from build123d import *

# Parameters (mm, degrees)
SKETCH_1_R               = 49
SKETCH_1_R_2             = 43
EXTRUDE_1_DEPTH          = 7.9
SKETCH_3_R               = 49
SKETCH_3_R_2             = 40.2
EXTRUDE_3_DEPTH          = 2
HOLE_WIZARD_M3_1_D       = 2.5
PATTERN_CIRCULAR_1_COUNT = 12


with BuildPart() as part:
    # 草图1 → 凸台-拉伸1 (new body)
    with BuildSketch(Plane.XY):
        Circle(SKETCH_1_R)
        Circle(SKETCH_1_R_2, mode=Mode.SUBTRACT)
    extrude(amount=EXTRUDE_1_DEPTH)

    # 草图3 → 凸台-拉伸3 (add)
    with BuildSketch(Plane.XY.offset(7.9)):
        Circle(SKETCH_3_R)
        Circle(SKETCH_3_R_2, mode=Mode.SUBTRACT)
    extrude(amount=EXTRUDE_3_DEPTH)

    # M3 螺纹孔1 (through all)
    with Locations(Plane(origin=(0, 0, 0), x_dir=(-1, 0, 0), z_dir=(0, 0, -1))):
        with Locations((0, 46)):
            hole_wizard_m3_1 = Hole(HOLE_WIZARD_M3_1_D / 2)

    # 阵列(圆周)1: M3 螺纹孔1 ×12 about axis
    pattern_circular_1_axis = Axis((0, 0, 0), (0, 0, 1))
    for i in range(1, PATTERN_CIRCULAR_1_COUNT):
        add(hole_wizard_m3_1.rotate(pattern_circular_1_axis, i * 360 / PATTERN_CIRCULAR_1_COUNT), mode=Mode.SUBTRACT)


solid = part.part
Geometry check sheet. Reference: the model listing, model coordinates, mm. A direction names the side the tool comes from. Round coordinates to 2 decimals unless told otherwise and drop trailing zeros. Order: outer loops, then holes, each group sorted by start corner. A loop starts at its lowest first (then second) coordinate and runs counter-clockwise, first axis right, second up. Notation, with made-up numbers: M -1.75,66 L 56.25,66 A22 cw 56.25,91 Z; hole C 45,-6.5 d3. An arc over 180 degrees is marked long. Answer in a Markdown table with one row per item. Add a question column.
Item 1: Material ranges on L1, parallel to Y at x = 0, z = 2.5; L2, parallel to Y at x = -1, z = 4.75; L3, parallel to X at y = 45, z = 4.75, recorded low to high. Write a range as [from, to].
Item 2: Sectioned sample at C-C, the plane y = -27. Enter the section's corners in (x, z), plus the area to 3 significant figures.
Item 3: Set-up check for faces 1 (the face through (-5.598, 42.634, 3.895)), 2 (the face through (24.11, -39.26, 5.02)): record each of +Z, -Z, +X, -X, +Y, -Y from which the full face is reachable in a straight line by a thin tool's end or side.
Item 4: Draft check along X on faces 3 (the face through (-0.16, 47.24, 5.02)), 4 (the face through (26.34, 41.32, 4.88)), 5 (the face through (-3.9, 40.2, 9.9)). Enter one of: released by +X, released by -X, zero draft, split by the parting line, or undercut.
Item 5: Sectioned sample at D-D, the plane x = -15.5. Enter the section's corners in (y, z), plus the area to 3 significant figures.
Item 6: Sectioned sample at A-A, the plane y = 0. Enter the section's corners in (x, z), plus the area to 3 significant figures.
Item 7: Depth check by flat-ended pin: pin 1 Ø2 at (x, y) = (0, 46) entering from -Z; pin 2 Ø1.5 at (x, z) = (28, 7.5) entering from +Y. Enter the tip coordinate at first touch or a pass-through.
Filled in:
| question | item | result |
|---|---|---|
| 1 | L1 | y = [-49, -47.25], [-44.75, -43], [43, 44.75], [47.25, 49] |
| 1 | L2 | y = [-48.99, -46.75], [-45.25, -42.99], [42.99, 45.25], [46.75, 48.99] |
| 1 | L3 | x = [-19.39, -0.75], [0.75, 19.39] |
| 2 | outline | M -40.89,0 L -33.47,0 L -33.47,7.9 L -29.78,7.9 L -29.78,9.9 L -40.89,9.9 Z; M 29.78,7.9 L 33.47,7.9 L 33.47,0 L 40.89,0 L 40.89,9.9 L 29.78,9.9 Z |
| 2 | area | 162 mm² |
| 3 | face 1 | -Z |
| 3 | face 2 | +Z, -Z |
| 4 | face 3 | undercut |
| 4 | face 4 | split by the parting line |
| 4 | face 5 | zero draft |
| 5 | outline | M -46.48,0 L -40.11,0 L -40.11,7.9 L -37.09,7.9 L -37.09,9.9 L -46.48,9.9 Z; M 37.09,7.9 L 40.11,7.9 L 40.11,0 L 46.48,0 L 46.48,9.9 L 37.09,9.9 Z |
| 5 | area | 138 mm² |
| 6 | outline | M -49,0 L -47.25,0 L -47.25,9.9 L -49,9.9 Z; M -44.75,0 L -43,0 L -43,7.9 L -40.2,7.9 L -40.2,9.9 L -44.75,9.9 Z; M 40.2,7.9 L 43,7.9 L 43,0 L 44.75,0 L 44.75,9.9 L 40.2,9.9 Z; M 47.25,0 L 49,0 L 49,9.9 L 47.25,9.9 Z |
| 6 | area | 80.5 mm² |
| 7 | pin 1 | passes through |
| 7 | pin 2 | stops at y = 40.72 |
